Here's the drawing with two shaded views (mm, measured from the low corner). I have some questions. A direction names the side the tool comes from. Give positions to 0.01 mm unless a question says otherwise; leave off trailing zeros. Write each loop counter-clockwise with the first axis right and the second up, starting at its lowest first coordinate (ties: lowest second). Pieces come first, ordered by that corner, then holes. Notation, with made-up numbers: (-11, -10) - (48, -10) arc R28 ccw to (48, 25) - close; hole circle Ø11 at (20, 2.5). An arc over 180 degrees is marked (long way). Answer as a JSON object with one key per item and string values. Group by question number.
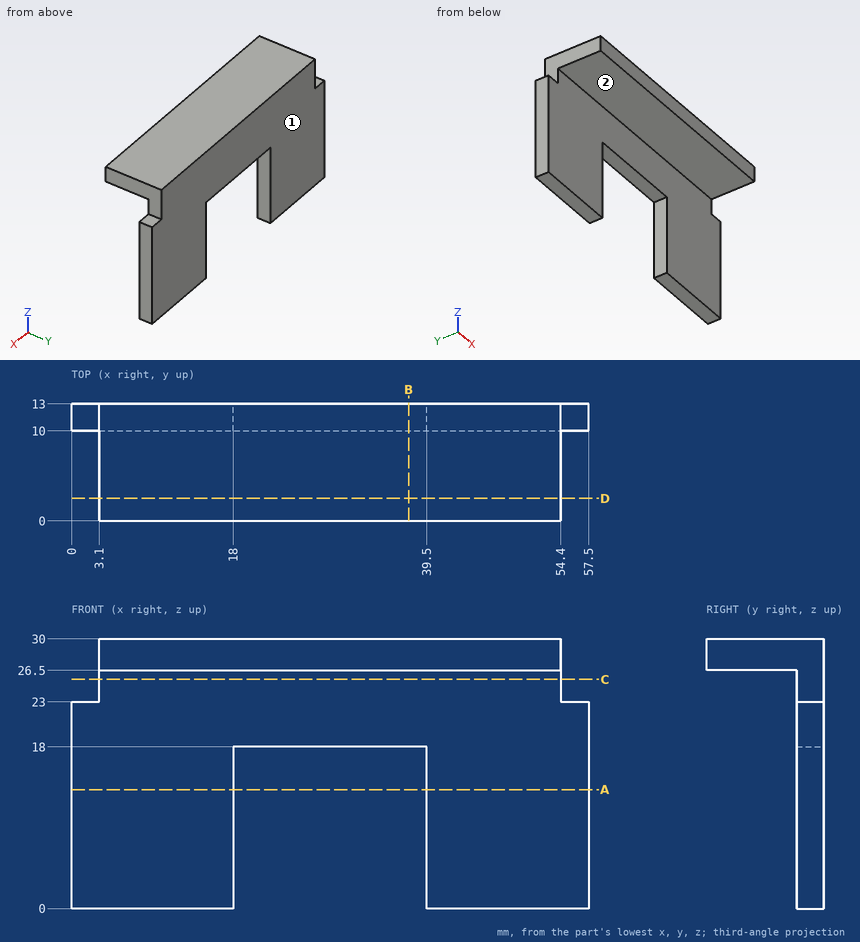
(1) I want a section at D-D, the plane y = 2.5. Please give me the cut outline in (x, z).
(2) I want a section at C-C, the plane z = 25.5. Please give me the cut outline in (x, y), and give its area (3 significant figures).
(3) For the marked faces 1 and 2, which set-ups out of +Z, -Z, +X, -X, +Y, -Y let a thin tool reach every point of the face, with its end or its side?
(4) I want a section at A-A, the plane z = 13.25. Please give me the cut outline in (x, y), and give its area (3 significant figures).
(5) I want a section at B-B, the plane x = 37.5. Please give me the cut outline in (y, z).
(6) Will these pins go through, and if not, where does the flat tip stop? P1, Ø1, axis at x = 13, z = 16, coming from the -Y side; P2, Ø3.5, axis at x = 1, y = 11, coming from the +Z side; P3, Ø8, axis at x = 27, z = 13, coming from the -Y side; P4, Ø5.5, axis at y = 7, z = 27.5, coming from the +X side.
(7) I need wall thicknesses on L1, parallel to X at y = 11.25, z = 17; L2, parallel to Z at x = 45, y = 9; L3, parallel to Y at x = 41, z = 3.75. Which ranges of each line are inside material? Lowest first, please.
Entries:
{
 "1": {"outline": "(3.1, 26.5) - (54.4, 26.5) - (54.4, 30) - (3.1, 30) - close"},
 "2": {"outline": "(3.1, 10) - (54.4, 10) - (54.4, 13) - (3.1, 13) - close", "area": "154 mm^2"},
 "3": {"face 1": "+Z, -Z, +X, -X, +Y", "face 2": "-Z, +X, -X, -Y"},
 "4": {"outline": "(0, 10) - (18, 10) - (18, 13) - (0, 13) - close; (39.5, 10) - (57.5, 10) - (57.5, 13) - (39.5, 13) - close", "area": "108 mm^2"},
 "5": {"outline": "(0, 26.5) - (10, 26.5) - (10, 18) - (13, 18) - (13, 30) - (0, 30) - close"},
 "6": {"P1": "y = 10", "P2": "z = 23", "P3": "through", "P4": "x = 54.4"},
 "7": {"L1": "0 to 18, 39.5 to 57.5", "L2": "26.5 to 30", "L3": "10 to 13"}
}
